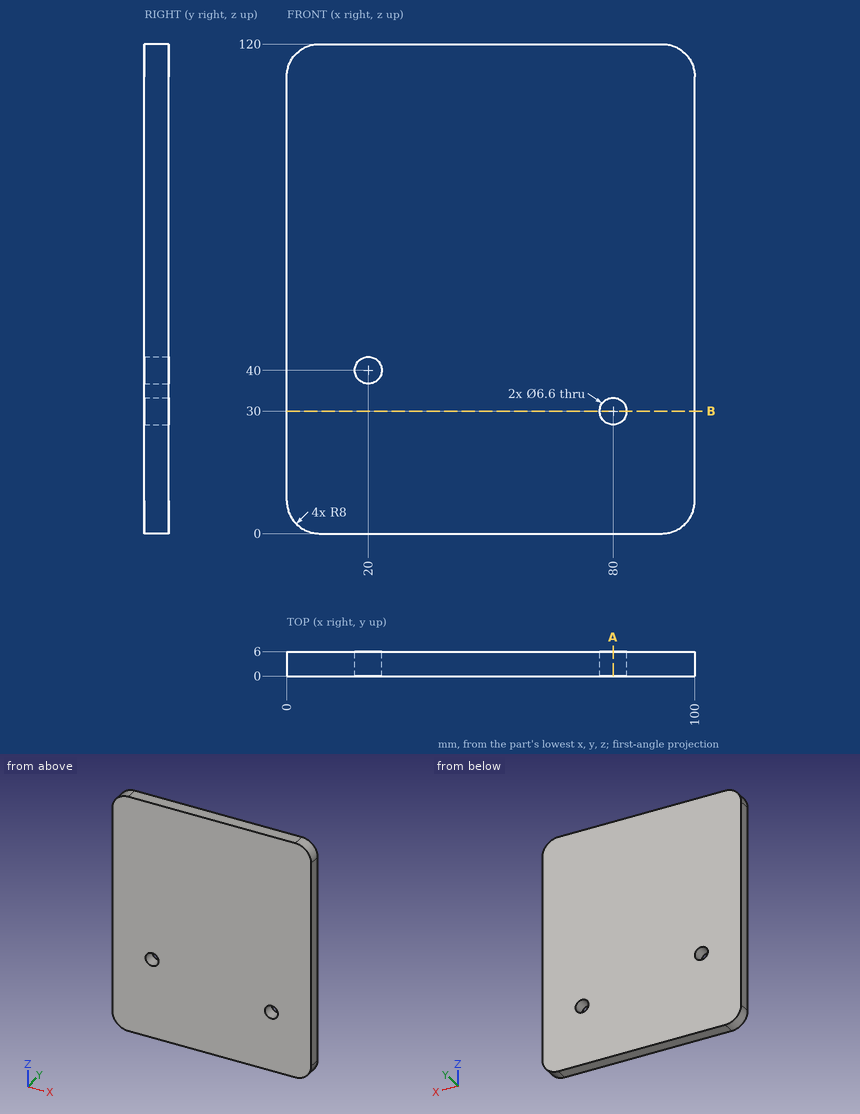
Could you check a few things on this drawing? It's one solid part, dimensions in mm from its lowest x, y, z. Give positions to 0.01 mm unless a question says otherwise; leave off trailing zeros. Order: outer loops, then holes, each group sorted by start corner. A loop starts at its lowest first (then second) coordinate and runs counter-clockwise, first axis right, second up. Notation, with made-up numbers: (8, 15.5) -> (38, 15.5) arc R8 cw to (38, 30.5) -> close; hole circle Ø6 at (61, 77.25). An arc over 180 degrees is marked (long way). Answer in a Markdown table with one row per item. Add a question column.
Item 1: Imagine slicing it at A-A (x = 80). List the corners of the cut face in (y, z) for me, and give its area (3 significant figures).
Item 2: Please list where these lines run through material, in increasing order: probe 1 along Z at (x, y) = (20, 2.75); probe 2 along Z at (x, y) = (80, 4.7); probe 3 along X at (y, z) = (4.3, 31).
Item 3: I'm going to push a flat-ended pin straight in: P1, Ø5.5, axis at x = 80, z = 30, coming from the +Y side. Where does the tip first touch, or does it pass through?
Item 4: Imagine slicing it at B-B (z = 30). List the corners of the cut face in (x, y) for me.
Result:
| question | item | result |
|---|---|---|
| 1 | outline | (0, 0) -> (6, 0) -> (6, 26.7) -> (0, 26.7) -> close; (0, 33.3) -> (6, 33.3) -> (6, 120) -> (0, 120) -> close |
| 1 | area | 680 mm2 |
| 2 | probe 1 | 0 to 36.7, 43.3 to 120 |
| 2 | probe 2 | 0 to 26.7, 33.3 to 120 |
| 2 | probe 3 | 0 to 76.86, 83.14 to 100 |
| 3 | P1 | through |
| 4 | outline | (0, 0) -> (76.7, 0) -> (76.7, 6) -> (0, 6) -> close; (83.3, 0) -> (100, 0) -> (100, 6) -> (83.3, 6) -> close |
